Can you work these out from the model? Positions are in its coordinate system, mm. A direction names the side the tool comes from. Round coordinates to 2 decimals unless told otherwise and drop trailing zeros. Write each loop counter-clockwise with the first axis right and the second up, starting at its lowest first coordinate (ties: lowest second). Pieces come first, ordered by that corner, then holes. Notation, with made-up numbers: (61.25, 4.5) -> (102.25, 4.5) arc R15 ccw to (102.25, 31.5) -> close; hole circle Ø9 at (-36, -4). An arc over 180 degrees is marked (long way). Write item = value, one per line. Start each with the question number.
1) Imagine slicing it at C-C, the plane z = 29. Please give me the cut outline in (x, y).
2) Imagine slicing it at B-B, the plane y = 0. Please give me the cut outline in (x, z).
3) I'm going to push flat-ended pins straight in: pin 1 (6 mm diameter, centred on x = 615.5, z = 68.5, fed in from +Y); pin 2 (10 mm diameter, centred on x = 876, z = 83, fed in from -Y); pin 3 (4 mm diameter, centred on y = -32.5, z = 197, fed in from -X). Where does each tip first touch, or does it pass through?
4) Imagine slicing it at D-D, the plane y = 159. Please give me the cut outline in (x, z).
5) If I drill on line 1 (Y direction, x = -25, z = 222); line 2 (X direction, y = 65, z = 131.5); line 3 (X direction, y = 13, z = 191), over which ranges is the centre line in solid material (lowest first)?
6) Thinking about a two-plate mould opening in Y: for faces 6 (the face through (1295.4, -40, 105)), 7 (the face through (90, 101.6, 97)), 8 (the face through (23.054, 15.259, 6.439)), which applies, +Y half, -Y half, draft (parallel to the pull), parting line (faces both ways), or undercut?
7) Imagine slicing it at A-A, the plane x = -25.4. Please give me the cut outline in (y, z), then the cut area to 3 significant figures.
8) For faces 1 (the face through (919.62, 138.34, 112.7)), 2 (the face through (90, -101.6, 97)), 3 (the face through (400.83, 242.44, 112.7)), 4 (the face through (37, 1, 12.7)), 5 (the face through (1215, -181, 215.9)), which set-ups out of +Z, -Z, +X, -X, +Y, -Y let a thin tool reach every point of the face, with its end or its side?
from build123d import *

# Parameters (mm, degrees)
SKETCH1_W           = 203.2
SKETCH1_H           = 203.2
BOSS_EXTRUDE1_DEPTH = 228.6
CUT_EXTRUDE1_DEPTH  = 228.6
SKETCH3_R           = 50.8
CUT_EXTRUDE2_DEPTH  = 271.005703643
BOSS_EXTRUDE2_DEPTH = 228.6
CUT_EXTRUDE3_DEPTH  = 1278.174091308
SKETCH7_R           = 50.8
CUT_EXTRUDE4_DEPTH  = 1373.616617817
SKETCH8_R           = 25.4
CUT_EXTRUDE5_DEPTH  = 1373.616617817


with BuildPart() as part:
    # Sketch1 → Boss-Extrude1 (new body)
    with BuildSketch(Plane.XY):
        Rectangle(SKETCH1_W, SKETCH1_H)
    extrude(amount=BOSS_EXTRUDE1_DEPTH)

    # Sketch2 → Cut-Extrude1 (cut)
    with BuildSketch(Plane(origin=(0, 101.6, 0), x_dir=(1, 0, 0), z_dir=(0, 1, 0))):
        Polygon((-88.9, -12.7), (-131.920098672, -12.7), (-131.920098672, -215.9), (-88.9, -215.9), (88.9, -215.9), (88.9, -12.7), align=None)
    extrude(amount=-CUT_EXTRUDE1_DEPTH, mode=Mode.SUBTRACT)

    # Sketch3 → Cut-Extrude2 (cut, through all)
    with BuildSketch(Plane.XY.offset(228.6)):
        with Locations((-25.4, 0)):
            Circle(SKETCH3_R)
    extrude(amount=-CUT_EXTRUDE2_DEPTH, mode=Mode.SUBTRACT)

    # Sketch5 → Boss-Extrude2 (add)
    with BuildSketch(Plane.XY):
        with BuildLine():
            Line((101.6, 101.6), (708.554663443, 387.282081105))
            ThreePointArc((708.554663443, 387.282081105), (735.661628292, 391.823256752), (761.166531666, 381.580711976))
            Line((761.166531666, 381.580711976), (1295.4, -29.464807141))
            Line((1295.4, -29.464807141), (1295.4, -232.664807141))
            Line((1295.4, -232.664807141), (1092.2, -232.664807141))
            Line((1092.2, -232.664807141), (1092.2, -29.464807141))
            Line((1092.2, -29.464807141), (742.133450583, 310.915917798))
            ThreePointArc((742.133450583, 310.915917798), (726.614813955, 318.010811429), (710.108636303, 313.685109437))
            Line((710.108636303, 313.685109437), (101.6, -101.6))
            Line((101.6, -101.6), (101.6, 101.6))
        make_face()
    extrude(amount=BOSS_EXTRUDE2_DEPTH)

    # Sketch6 → Cut-Extrude3 (cut, through all)
    with BuildSketch(Plane.ZY.offset(-1092.2)):
        Polygon((12.7, -219.964807141), (12.7, -266.729426715), (215.9, -266.729426715), (215.9, -219.964807141), (215.9, -42.164807141), (12.7, -42.164807141), align=None)
    extrude(amount=-CUT_EXTRUDE3_DEPTH, mode=Mode.SUBTRACT)

    # Sketch7 → Cut-Extrude4 (cut, through all)
    with BuildSketch(Plane.XY.offset(228.6)):
        with Locations((1193.8, -131.064807141)):
            Circle(SKETCH7_R)
    extrude(amount=-CUT_EXTRUDE4_DEPTH, mode=Mode.SUBTRACT)

    # Sketch8 → Cut-Extrude5 (cut, through all)
    with BuildSketch(Plane.XY.offset(228.6)):
        with Locations((728.615646145, 349.569241459)):
            Circle(SKETCH8_R)
    extrude(amount=-CUT_EXTRUDE5_DEPTH, mode=Mode.SUBTRACT)


solid = part.part
Reported:
q1.outline = (88.9, -101.6) -> (101.6, -101.6) -> (710.11, 313.69) arc R25.4 cw to (742.13, 310.92) -> (1092.2, -29.46) -> (1092.2, -42.16) -> (1295.4, -42.16) -> (1295.4, -29.46) -> (761.17, 381.58) arc R50.8 ccw to (708.55, 387.28) -> (101.6, 101.6) -> (88.9, 101.6) -> close; hole circle Ø50.8 at (728.62, 349.57)
q2.outline = (-101.6, 0) -> (-76.2, 0) -> (-76.2, 12.7) -> (-101.6, 12.7) -> close; (-101.6, 215.9) -> (-76.2, 215.9) -> (-76.2, 228.6) -> (-101.6, 228.6) -> close; (25.4, 0) -> (250.47, 0) -> (250.47, 228.6) -> (25.4, 228.6) -> (25.4, 215.9) -> (88.9, 215.9) -> (88.9, 12.7) -> (25.4, 12.7) -> close; (1061.9, 0) -> (1257.1, 0) -> (1257.1, 228.6) -> (1061.9, 228.6) -> close
q3.pin_1 = 344.9
q3.pin_2 = 175.89
q3.pin_3 = 88.9
q4.outline = (223.55, 0) -> (483.45, 0) -> (483.45, 228.6) -> (223.55, 228.6) -> close; (898.37, 0) -> (1050.45, 0) -> (1050.45, 228.6) -> (898.37, 228.6) -> close
q5.line_1 = -101.6 to -50.8, 50.8 to 101.6
q5.line_2 = 88.9 to 345.72, 995.05 to 1172.62
q5.line_3 = 88.9 to 269.52, 1048.53 to 1240.21
q6.face_6 = draft
q6.face_7 = +Y half
q6.face_8 = undercut
q7.outline = (-101.6, 0) -> (-50.8, 0) -> (-50.8, 12.7) -> (-101.6, 12.7) -> close; (-101.6, 215.9) -> (-50.8, 215.9) -> (-50.8, 228.6) -> (-101.6, 228.6) -> close; (50.8, 0) -> (101.6, 0) -> (101.6, 12.7) -> (50.8, 12.7) -> close; (50.8, 215.9) -> (101.6, 215.9) -> (101.6, 228.6) -> (50.8, 228.6) -> close
q7.area = 2,580 mm²
q8.face_1 = +Z, -Z, -Y
q8.face_2 = +Z, -Z, -X, -Y
q8.face_3 = +Z, -Z, -X, +Y
q8.face_4 = -X, +Y, -Y
q8.face_5 = +X, -Y
